from build123d import *

# Parameters (mm, degrees)
SKETCH1_R                    = 180
BOSS_EXTRUDE1_DEPTH          = 50
BOSS_EXTRUDE2_DEPTH          = 32.148542
SKETCH3_R                    = 12.5
CUT_EXTRUDE1_DEPTH           = 5
M12_TAPPED_HOLE1_D           = 10.2
M12_TAPPED_HOLE1_DEPTH       = 17.5
M12_TAPPED_HOLE1_CSINK_D     = 12.05
M12_TAPPED_HOLE1_CSINK_ANGLE = 90
M12_TAPPED_HOLE1_TIP         = 3.064389157
SKETCH8_R                    = 10
BOSS_EXTRUDE3_DEPTH          = 5
SKETCH9_R                    = 7.5
SKETCH9_R_2                  = 5
BOSS_EXTRUDE4_DEPTH          = 5


# Read off the part's stored shape, not the designer's step: M18 Machine Threads Stud1, M18 Machine Threads Stud2
with BuildPart() as part:
    # Sketch1 → Boss-Extrude1 (new body)
    with BuildSketch(Plane(origin=(0, 0, 0), x_dir=(1, 0, 0), z_dir=(0, 1, 0))):
        with Locations(Location((0, 0, 0), (0, 0, 270))):
            Circle(SKETCH1_R)
    extrude(amount=BOSS_EXTRUDE1_DEPTH)

    # Sketch2 → Boss-Extrude2 (add)
    with BuildSketch(Plane(origin=(0, 50, 0), x_dir=(1, 0, 0), z_dir=(0, 1, 0))):
        Polygon((-84.548207039, -115.101573323), (-39.951504434, -74.962638151), (-93.470084664, -15.500368011), (-138.066787269, -55.639303183), align=None)
        Polygon((-40.744531967, -124.452472721), (36.749910483, -144.317300669), (51.648531443, -86.196468831), (-25.845911006, -66.331640884), align=None)
        Polygon((126.114531486, 92.960164639), (69.721759674, 149.703933348), (27.163933142, 107.409354489), (83.556704954, 50.66558578), align=None)
    extrude(amount=BOSS_EXTRUDE2_DEPTH)

    # Sketch3 → Cut-Extrude1 (cut)
    with BuildSketch(Plane(origin=(0, 50, 0), x_dir=(1, 0, 0), z_dir=(0, 1, 0))):
        with Locations(Location((-35.5, 59.3, 0), (0, 0, 270))):
            Circle(SKETCH3_R)
        with Locations(Location((19.854, -49.141, 0), (0, 0, 270))):
            Circle(SKETCH3_R)
    extrude(amount=-CUT_EXTRUDE1_DEPTH, mode=Mode.SUBTRACT)

    # M12 Tapped Hole1
    with Locations(Plane(origin=(0, 50, 0), x_dir=(1, 0, 0), z_dir=(0, 1, 0))):
        with Locations((35.5, 59.3), (-45.899, -26.5)):
            CounterSinkHole(M12_TAPPED_HOLE1_D / 2, M12_TAPPED_HOLE1_CSINK_D / 2, depth=M12_TAPPED_HOLE1_DEPTH, counter_sink_angle=M12_TAPPED_HOLE1_CSINK_ANGLE)
            with Locations((0, 0, -(M12_TAPPED_HOLE1_DEPTH + M12_TAPPED_HOLE1_TIP / 2))):  # 118° drill point
                Cone(0, M12_TAPPED_HOLE1_D / 2, M12_TAPPED_HOLE1_TIP, mode=Mode.SUBTRACT)

    # Sketch8 → Boss-Extrude3 (add)
    with BuildSketch(Plane(origin=(0, 45, 0), x_dir=(1, 0, 0), z_dir=(0, 1, 0))):
        with Locations(Location((-35.5, 59.3, 0), (0, 0, 270))):
            Circle(SKETCH8_R)
        with Locations(Location((19.854, -49.141, 0), (0, 0, 270))):
            Circle(SKETCH8_R)
    extrude(amount=BOSS_EXTRUDE3_DEPTH)

    # Sketch9 → Boss-Extrude4 (add)
    # profile 1 of 2: a face of its own
    with BuildSketch(Plane(origin=(0, 50, 0), x_dir=(1, 0, 0), z_dir=(0, 1, 0))):
        with Locations(Location((-35.5, 59.3, 0), (0, 0, 270))):
            Circle(SKETCH9_R)
        with Locations(Location((-35.5, 59.3, 0), (0, 0, 270))):
            Circle(SKETCH9_R_2, mode=Mode.SUBTRACT)
    # profile 2 of 2: a face of its own
    with BuildSketch(Plane(origin=(0, 50, 0), x_dir=(1, 0, 0), z_dir=(0, 1, 0))):
        with Locations(Location((19.854, -49.141, 0), (0, 0, 270))):
            Circle(SKETCH9_R)
        with Locations(Location((19.854, -49.141, 0), (0, 0, 270))):
            Circle(SKETCH9_R_2, mode=Mode.SUBTRACT)
    extrude(amount=BOSS_EXTRUDE4_DEPTH)

    # M18 Machine Threads Stud1 outline → M18 Machine Threads Stud1 (revolve, cut)
    with BuildSketch(Plane(origin=(-35.5, 0, -59.3), x_dir=(1, 0, 0), z_dir=(0, 0, 1))):
        Polygon((9, 48.626), (9, 45), (10, 45), (10, 50), (7.626, 50), align=None)
    revolve(axis=Axis((-35.5, 0, -59.3), (0, 1, 0)), mode=Mode.SUBTRACT)

    # M18 Machine Threads Stud2 outline → M18 Machine Threads Stud2 (revolve, cut)
    with BuildSketch(Plane(origin=(19.854, 0, 49.141), x_dir=(1, 0, 0), z_dir=(0, 0, 1))):
        Polygon((9, 48.626), (9, 45), (10, 45), (10, 50), (7.626, 50), align=None)
    revolve(axis=Axis((19.854, 0, 49.141), (0, 1, 0)), mode=Mode.SUBTRACT)


solid = part.part
Geometry: final body of the model. Coordinates: model frame, mm. A direction names the side the tool comes from. Round coordinates to 2 decimals unless told otherwise and drop trailing zeros. Order: outer loops, then holes, each group sorted by start corner. A loop starts at its lowest first (then second) coordinate and runs counter-clockwise, first axis right, second up. Notation, with made-up numbers: (-7.75, 60.5) - (-2.75, 60.5) arc R22 ccw to (-2.75, 96.5) - close; hole circle Ø5 at (88, 51.25). An arc over 180 degrees is marked (long way). Write each question's results on one line, items separated by ' | '.
Item 1: Section A-A, the plane y = 64. Return the cut outline in (x, z).
Completed:
outline: (-138.07, 55.64) - (-93.47, 15.5) - (-39.95, 74.96) - (-84.55, 115.1) - close; (-40.74, 124.45) - (-25.85, 66.33) - (51.65, 86.2) - (36.75, 144.32) - close; (27.16, -107.41) - (69.72, -149.7) - (126.11, -92.96) - (83.56, -50.67) - close
Item 2: Mould query, pull axis Z, two halves, no side actions, for faces 4 (the cylindrical face through (-68.941, 24.65, 166.274)), 5 (the cylindrical face through (39.55, 40.67, -56.2)), 6 (the flat face through (-37, 55, -54)). Classes: pulls with the +Z half, pulls with the -Z half, needs draft (parallel to the pull), parting line crosses it, or undercut.
Completed:
face 4: parting line crosses it | face 5: undercut | face 6: needs draft
Item 3: Section C-C, the plane z = 0. Return the cut outline in (x, y), and give its area (3 significant figures).
Completed:
outline: (-180, 0) - (180, 0) - (180, 50) - (-180, 50) - close | area: 18,000 mm^2
Item 4: Section B-B, the plane x = 119. Return the cut outline in (y, z).
Completed:
outline: (0, -135.05) - (50, -135.05) - (50, -100.12) - (82.15, -100.12) - (82.15, -85.89) - (50, -85.89) - (50, 135.05) - (0, 135.05) - close
Item 5: Section D-D, the plane x = -35.5. Return the cut outline in (y, z).
Completed:
outline: (0, -176.46) - (50, -176.46) - (50, -71.8) - (45, -71.8) - (45, -68.3) - (48.63, -68.3) - (50, -66.93) - (50, -66.8) - (55, -66.8) - (55, -64.3) - (50, -64.3) - (50, -54.3) - (55, -54.3) - (55, -51.8) - (50, -51.8) - (50, -51.67) - (48.63, -50.3) - (45, -50.3) - (45, -46.8) - (50, -46.8) - (50, 103.99) - (82.15, 103.99) - (82.15, 125.8) - (50, 125.8) - (50, 176.46) - (0, 176.46) - close
Item 6: First-contact query: pin 1 Ø1 at (y, z) = (60.5, 111) entering from -X; pin 2 Ø3 at (x, z) = (100, 83) entering from -Y; pin 3 Ø7.5 at (x, z) = (22.5, 48) entering from +Y; pin 4 Ø4 at (x, y) = (28, 33) entering from -Z. Flat tips, straight axial feed; report the tip coordinate or a pass-through.
Completed:
pin 1: x = -88.69 | pin 2: y = 0 | pin 3: y = 55 | pin 4: z = -178.11
Item 7: Reachability of faces 1 (the cylindrical face through (-41.85, 40.67, 29.6)), 2 (the flat face through (-111.682, 65.849, 84.954)), 3 (the flat face through (-115.46, 65.85, 35.29)) from +Z, -Z, +X, -X, +Y, -Y: full face, straight path, thin tool, end or side. Return the list, or none.
Completed:
face 1: +Y | face 2: +Z, -X, +Y | face 3: -Z, -X, +Y
Item 8: Material intervals for line 1 along X through (y, z) = (51, -59); line 2 along X through (y, z) = (47.5, -66.5); line 3 along Y through (x, z) = (6, -74), sorted ascending. Write a range as [from, to].
Completed:
line 1: [-42.99, -40.49], [-30.51, -28.01], [75.27, 91.94] | line 2: [-167.27, -45.72], [-40.9, -30.1], [-25.28, 167.27] | line 3: [0, 50]
